```python
from build123d import *

# Parameters (mm, degrees)
SKETCH1_W                                      = 127
SKETCH1_H                                      = 12.7
BOSS_EXTRUDE1_DEPTH                            = 38.1
SKETCH3_R                                      = 4.445
CUT_EXTRUDE3_DEPTH                             = 2.54
CUT_EXTRUDE4_DEPTH                             = 13.208
CUT_EXTRUDE4_DEPTH_BACK                        = 13.208
SKETCH2_R                                      = 7.9756
SKETCH2_R_2                                    = 8.1026
SKETCH6_R                                      = 5.08
CUT_EXTRUDE5_DEPTH                             = 38.1
F_11_64_0_17188_DIAMETER_HOLE1_D               = 4.365752
F_11_64_0_17188_DIAMETER_HOLE1_DEPTH           = 25.4
F_11_64_0_17188_DIAMETER_HOLE1_TIP             = 1.311604225
F_11_64_0_17188_DIAMETER_HOLE1_ON_FACE_2_D     = 4.365752
F_11_64_0_17188_DIAMETER_HOLE1_ON_FACE_2_DEPTH = 25.4
F_11_64_0_17188_DIAMETER_HOLE1_ON_FACE_2_TIP   = 1.311604225
SKETCH9_R                                      = 2.54
CUT_EXTRUDE7_DEPTH                             = 11.43
SKETCH10_W                                     = 6.604
SKETCH10_H                                     = 9.398
CUT_EXTRUDE10_DEPTH                            = 76.134213245
CUT_EXTRUDE11_START                            = -11.43
SKETCH11_R                                     = 2.54
CUT_EXTRUDE11_DEPTH                            = 11.43


with BuildPart() as part:
    # Sketch1 → Boss-Extrude1 (new body)
    with BuildSketch(Plane(origin=(0, 0, 0), x_dir=(1, 0, 0), z_dir=(0, 1, 0))):
        with Locations((0, -6.35)):
            Rectangle(SKETCH1_W, SKETCH1_H)
    extrude(amount=BOSS_EXTRUDE1_DEPTH)

    # Sketch3 → Cut-Extrude3 (cut)
    with BuildSketch(Plane(origin=(0, 0, 0), x_dir=(-1, 0, 0), z_dir=(0, 0, -1))):
        with Locations((-58.039, 31.75)):
            Circle(SKETCH3_R)
        with Locations((-58.039, 6.35)):
            Circle(SKETCH3_R)
        with Locations((-31.009232106, 31.75)):
            Circle(SKETCH3_R)
        with Locations((-31.009232106, 6.35)):
            Circle(SKETCH3_R)
        with Locations((31.009232106, 31.75)):
            Circle(SKETCH3_R)
        with Locations((31.009232106, 6.35)):
            Circle(SKETCH3_R)
        with Locations((58.039, 31.75)):
            Circle(SKETCH3_R)
        with Locations((58.039, 6.35)):
            Circle(SKETCH3_R)
    extrude(amount=-CUT_EXTRUDE3_DEPTH, mode=Mode.SUBTRACT)

    # Sketch2 → Cut-Extrude4 (cut, two sides: drawn at the far end of the back side and taken through both)
    with BuildSketch(Plane(origin=(0, 19.05, 0), x_dir=(1, 0, 0), z_dir=(0, 1, 0)).offset(-CUT_EXTRUDE4_DEPTH_BACK)):
        with Locations((-44.45, -13.97)):
            Circle(SKETCH2_R)
        with Locations((44.45, -13.97)):
            Circle(SKETCH2_R_2)
    extrude(amount=CUT_EXTRUDE4_DEPTH + CUT_EXTRUDE4_DEPTH_BACK, mode=Mode.SUBTRACT)

    # Sketch6 → Cut-Extrude5 (cut)
    with BuildSketch(Plane(origin=(0, 38.1, 0), x_dir=(1, 0, 0), z_dir=(0, 1, 0))):
        with Locations((-44.45, -13.97)):
            Circle(SKETCH6_R)
        with Locations((44.45, -13.97)):
            Circle(SKETCH6_R)
    extrude(amount=-CUT_EXTRUDE5_DEPTH, mode=Mode.SUBTRACT)

    # 11/64 (0.17188) Diameter Hole1
    with Locations(Plane(origin=(58.039, 31.75, 0), x_dir=(-1, 0, 0), z_dir=(0, 0, -1))):
        with Locations((0, 0), (27.029767894, 0), (27.029767894, -25.4), (89.048232106, -25.4), (116.078, 0)):
            Hole(F_11_64_0_17188_DIAMETER_HOLE1_D / 2, depth=F_11_64_0_17188_DIAMETER_HOLE1_DEPTH)
            with Locations((0, 0, -(F_11_64_0_17188_DIAMETER_HOLE1_DEPTH + F_11_64_0_17188_DIAMETER_HOLE1_TIP / 2))):  # 118° drill point
                Cone(0, F_11_64_0_17188_DIAMETER_HOLE1_D / 2, F_11_64_0_17188_DIAMETER_HOLE1_TIP, mode=Mode.SUBTRACT)

    # 11/64 (0.17188) Diameter Hole1 on face 2
    with Locations(Plane(origin=(58.039, 6.35, 2.54), x_dir=(-1, 0, 0), z_dir=(0, 0, -1))):
        with Locations((0, 0), (89.048232106, 25.4), (116.078, 0)):
            Hole(F_11_64_0_17188_DIAMETER_HOLE1_ON_FACE_2_D / 2, depth=F_11_64_0_17188_DIAMETER_HOLE1_ON_FACE_2_DEPTH)
            with Locations((0, 0, -(F_11_64_0_17188_DIAMETER_HOLE1_ON_FACE_2_DEPTH + F_11_64_0_17188_DIAMETER_HOLE1_ON_FACE_2_TIP / 2))):  # 118° drill point
                Cone(0, F_11_64_0_17188_DIAMETER_HOLE1_ON_FACE_2_D / 2, F_11_64_0_17188_DIAMETER_HOLE1_ON_FACE_2_TIP, mode=Mode.SUBTRACT)

    # Sketch9 → Cut-Extrude7 (cut)
    with BuildSketch(Plane.ZY.offset(63.5)):
        with Locations((6.35, 19.05)):
            Circle(SKETCH9_R)
    extrude(amount=-CUT_EXTRUDE7_DEPTH, mode=Mode.SUBTRACT)

    # Sketch10 → Cut-Extrude10 (cut, through all)
    with BuildSketch(Plane.XY.offset(12.7)):
        with Locations((-56.895836127, 19.177)):
            Rectangle(SKETCH10_W, SKETCH10_H)
        with Locations((56.895836127, 19.177)):
            Rectangle(SKETCH10_W, SKETCH10_H)
    extrude(amount=-CUT_EXTRUDE10_DEPTH, mode=Mode.SUBTRACT)

    # Sketch11 → Cut-Extrude11 (cut)
    with BuildSketch(Plane(origin=(63.5, 0, 0), x_dir=(0, 0, -1), z_dir=(1, 0, 0)).offset(CUT_EXTRUDE11_START)):
        with Locations(Location((-6.35, 19.05, 0), (0, 0, 180))):
            Circle(SKETCH11_R)
    extrude(amount=CUT_EXTRUDE11_DEPTH, mode=Mode.SUBTRACT)


solid = part.part
```
Here's how the part is built. I have some questions about the finished solid (model axes, mm). A direction names the side the tool comes from. Round coordinates to 2 decimals unless told otherwise and drop trailing zeros. Order: outer loops, then holes, each group sorted by start corner. A loop starts at its lowest first (then second) coordinate and runs counter-clockwise, first axis right, second up. Notation, with made-up numbers: M 1,76 L 24,76 A31 ccw 24,106 Z; hole C 2,23.5 d11. An arc over 180 degrees is marked long. Answer in a Markdown table with one row per item.
Item 1: I'm going to push flat-ended pins straight in: pin 1 (5 mm diameter, centred on x = -58.039, y = 31.75, fed in from +Z); pin 2 (7 mm diameter, centred on x = 31.01, y = 31.75, fed in from -Z). Where does each tip first touch, or does it pass through?
A:
| item | result |
|---|---|
| pin 1 | stops at z = 12.7 |
| pin 2 | stops at z = 2.54 |
Item 2: Thinking about a two-plate mould opening in X: for faces 1 (the face through (44.54, 35.22, 8.89)), 2 (the face through (61.83, 16.53, 6.02)), 3 (the face through (52.07, 19, 6)), which applies, +X half, -X half, draft (parallel to the pull), parting line (faces both ways), or undercut?
A:
| item | result |
|---|---|
| face 1 | undercut |
| face 2 | draft |
| face 3 | +X half |
Item 3: For faces 4 (the face through (-35.249, 33.085, 1.252)), 5 (the face through (-57, 23.876, 6)), 6 (the face through (44, 32.258, 8)), which set-ups out of +Z, -Z, +X, -X, +Y, -Y let a thin tool reach every point of the face, with its end or its side?
A:
| item | result |
|---|---|
| face 4 | -Z |
| face 5 | +Z, -Z |
| face 6 | +Z |
Item 4: Imagine slicing it at B-B, the plane x = 47. Write out the boundary of the cut face in (y, z), and give its area (3 significant figures).
A:
| item | result |
|---|---|
| outline | M 0,0 L 38.1,0 L 38.1,9.58 L 32.26,9.58 L 32.26,6.28 L 5.84,6.28 L 5.84,9.58 L 0,9.58 Z |
| area | 278 mm2 |
Item 5: Imagine slicing it at A-A, the plane y = 19.05. State how many separate pieces and enclosed holes the cut face has, and give its area (3 significant figures).
A:
| item | result |
|---|---|
| separate pieces | 5 |
| enclosed holes | 0 |
| area | 1,230 mm2 |
Item 6: If I drill on L1, parallel to Y at x = -40, z = 7.5; L2, parallel to Y at x = 28.5, z = 1.75; L3, parallel to Y at x = 55, z = 9.5, over which ranges is the centre line in solid material (lowest first)? Write a range as from..to.
A:
| item | result |
|---|---|
| L1 | y = 0..5.84, 32.26..38.1 |
| L2 | y = 0..2.68, 10.02..28.08, 35.42..38.1 |
| L3 | y = 0..14.48, 23.88..38.1 |
